Work out the finished part from the listing and answer in its coordinate system (mm). Face numbers are marked on the shaded views. A direction names the side the tool comes from. Give positions to 0.01 mm unless a question says otherwise; leave off trailing zeros. Loops run counter-clockwise (first coordinate to the right, second up) from the corner with the lowest first, then second, coordinate; pieces in that order, holes last. Notation, with made-up numbers: M -31,-40 L 27,-40 A12 cw 27,-21 Z; hole C 75,-10.75 d6. An arc over 180 degrees is marked long. Use a Markdown table: item, result.
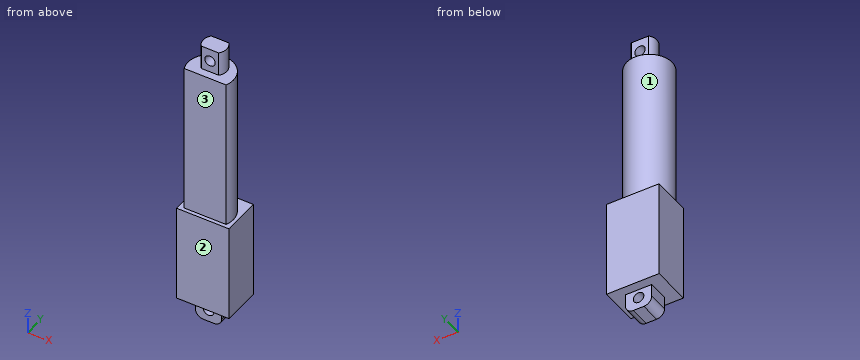
Autodesk Inventor part; units mm, degrees
ref_plane "YZ Plane" through (0, 0, 0) normal (1, 0, 0) x (0, 1, 0)
ref_plane "XZ Plane" through (0, 0, 0) normal (0, 1, 0) x (-1, 0, 0)
ref_plane "XY Plane" through (0, 0, 0) normal (0, 0, 1) x (1, 0, 0)
sketch "Sketch1" plane through (0, 0, 0) normal (0, 0, 1) x (1, 0, 0)
  line L0 (0, 0) -> (20, 0)
  line L1 (20, 0) -> (20, -14.8)
  line L2 (20, -14.8) -> (0, -14.8)
  line L3 (0, -14.8) -> (0, 0)
  dimension "d0" = 20
  dimension "d1" = 14.8
extrude "Extrusion1" add sketch "Sketch1" along normal blind 37.4
sketch "Sketch2" plane through (0, 0, 37.4) normal (0, 0, 1) x (1, 0, 0)
  line L0 (0, 0) -> (0, -14.8)
  line L1 (20, 0) -> (0, 0)
  line L2 (2, -13.4) -> (18, -13.4)
  arc A0 (18, -13.4) -> (2, -13.4) centre (10, -10.0667) ccw
  point P0 (10, -7.4)
  point P1 (10, -13.4)
extrude "Extrusion2" add sketch "Sketch2" along normal blind 58.1
sketch "Sketch3" plane through (0, 0, 95.5) normal (0, 0, 1) x (1, 0, 0)
  arc A0 (18, -13.4) -> (2, -13.4) centre (10, -10.0667) ccw
  line L0 (2, -13.4) -> (18, -13.4)
  line L1 (2, -13.4) -> (2, -13.4)
  line L2 (2, -13.4) -> (2, -13.4) construction
  line L3 (10, -13.4) -> (22, -13.4) construction
  line L4 (18, -13.4) -> (2, -13.4)
  line L5 (0, -14.8) -> (20, -14.8)
  line L6 (6.6913, -4.35) -> (13.3087, -4.35)
  line L7 (6.6913, -10.45) -> (13.3087, -10.45)
  arc A1 (6.6913, -4.35) -> (6.6913, -10.45) centre (10, -7.4) ccw
  arc A2 (13.3087, -10.45) -> (13.3087, -4.35) centre (10, -7.4) ccw
  point P0 (0, 0)
  dimension "d12" = 90
extrude "Extrusion3" add sketch "Sketch3" along normal blind 9.3 contours L6 A2 L7 A1
sketch "Sketch4" plane through (6.6913, -4.35, 95.5) normal (0, 1, 0) x (1, 0, 0)
  circle A0 centre (3.3087, -4.5) radius 2
  line L0 (-5.358, 0) -> (11.9754, 0)
  point P0 (-6.6913, 95.5)
  point P1 (11.3087, 0)
  point P2 (-4.6913, 0)
  dimension "d21" = 4
  dimension "d22" = 4.5
extrude "Extrusion4" cut sketch "Sketch4" against normal through all
sketch "Sketch5" plane through (0, 0, 0) normal (0, 0, -1) x (-1, 0, 0)
  line L0 (-15, -3.5) -> (-5, -3.5)
  line L1 (-5, -3.5) -> (-5, -11.3)
  line L2 (-5, -11.3) -> (-15, -11.3)
  line L3 (-15, -11.3) -> (-15, -3.5)
  line L4 (-15, -3.5) -> (-5, -11.3) construction
  line L5 (-5, -3.5) -> (-15, -11.3) construction
  line L6 (-20, 0) -> (0, 0)
  line L7 (0, -14.8) -> (-20, -14.8)
  line L8 (0, 0) -> (0, -14.8)
  line L9 (-20, 0) -> (0, 0)
  line L10 (-20, -14.8) -> (-20, 0)
  point P0 (-10, -7.4)
  point P1 (0, -7.4)
  point P2 (-10, -7.4)
  dimension "d25" = 7.8
  dimension "d26" = 10
  dimension "d27" = 10
extrude "Extrusion5" add sketch "Sketch5" along normal blind 7.8 contours L0 L1 L2 L3
sketch "Sketch6" plane through (5, -3.5, 0) normal (0, 1, 0) x (1, 0, 0)
  circle A0 centre (5, 3.3) radius 2
  line L0 (0, 7.8) -> (10, 7.8)
  line L1 (0, 0) -> (0, 7.8)
  point P0 (-5, 0)
  point P1 (5, 7.8)
  dimension "d30" = 4
  dimension "d31" = 4.5
  dimension "d32" = 5
extrude "Extrusion6" cut sketch "Sketch6" against normal through all
fillet "Fillet1" radius 3 2 edges at (15, -7.4, -7.8) (5, -7.4, -7.8)
properties part number "actuator"
(1) A cutting plane is placed at A-A (z = -3.3). Write down the section's boundary in (x, y).
Entries:
| item | result |
|---|---|
| outline | M 5,-11.3 L 8,-11.3 L 8,-3.5 L 5,-3.5 Z; M 12,-11.3 L 15,-11.3 L 15,-3.5 L 12,-3.5 Z |
(2) A cutting plane is placed at B-B (x = 10). Write down the section's boundary in (y, z), and give its area (3 significant figures).
Entries:
| item | result |
|---|---|
| outline | M -14.8,0 L -11.3,0 L -11.3,-1.3 L -3.5,-1.3 L -3.5,0 L 0,0 L 0,37.4 L -1.4,37.4 L -1.4,95.5 L -4.35,95.5 L -4.35,98 L -10.45,98 L -10.45,95.5 L -13.4,95.5 L -13.4,37.4 L -14.8,37.4 Z; M -11.3,-7.8 L -3.5,-7.8 L -3.5,-5.3 L -11.3,-5.3 Z; M -10.45,102 L -4.35,102 L -4.35,104.8 L -10.45,104.8 Z |
| area | 1,310 mm² |
(3) Which of the six approach directions +Z, -Z, +X, -X, +Y, -Y give full straight-line access (tool end or side, diameter ignored) to the marked faces 1, 2 and 3?
Entries:
| item | result |
|---|---|
| face 1 | +Z |
| face 2 | +Z, -Z, +X, -X, -Y |
| face 3 | +Z, +X, -X, -Y |
(4) A cutting plane is placed at C-C (y = -7.25). Write down the section's boundary in (x, z).
Entries:
| item | result |
|---|---|
| outline | M 0,0 L 5,0 L 5,-4.8 A3 ccw 8,-7.8 L 12,-7.8 A3 ccw 15,-4.8 L 15,0 L 20,0 L 20,37.4 L 18.2,37.4 L 18.2,95.5 L 14.5,95.5 L 14.5,104.8 L 5.5,104.8 L 5.5,95.5 L 1.8,95.5 L 1.8,37.4 L 0,37.4 Z; hole C 10,-3.3 d4; hole C 10,100 d4 |
(5) Consider probe 1 along Z at (x, y) = (10, -7); probe 2 along X at (y, z) = (-5.5, -3.3); probe 3 along Z at (x, y) = (4.75, -6.5). Determine where each line is inside the solid, lowest interval first. Write a range as [from, to].
Entries:
| item | result |
|---|---|
| probe 1 | z = [-7.8, -5.3], [-1.3, 98], [102, 104.8] |
| probe 2 | x = [5, 8], [12, 15] |
| probe 3 | z = [0, 95.5] |
(6) A cutting plane is placed at D-D (z = 100). Write down the section's boundary in (x, y).
Entries:
| item | result |
|---|---|
| outline | M 6.69,-10.45 L 8,-10.45 L 8,-4.35 L 6.69,-4.35 A4.5 ccw Z; M 12,-10.45 L 13.31,-10.45 A4.5 ccw 13.31,-4.35 L 12,-4.35 Z |
(7) Given P1, Ø3, axis at x = 2, y = -5, coming from the -Z side; P2, Ø5.5, axis at x = 9, z = 99, coming from the +Y side; P3, Ø4, axis at x = 15.5, z = 87.5, coming from the -Y side, each flat-ended and moving along its own axis, determine where each tip first touches the part or whether it passes through.
Entries:
| item | result |
|---|---|
| P1 | stops at z = 0 |
| P2 | stops at y = -4.35 |
| P3 | stops at y = -13.4 |
